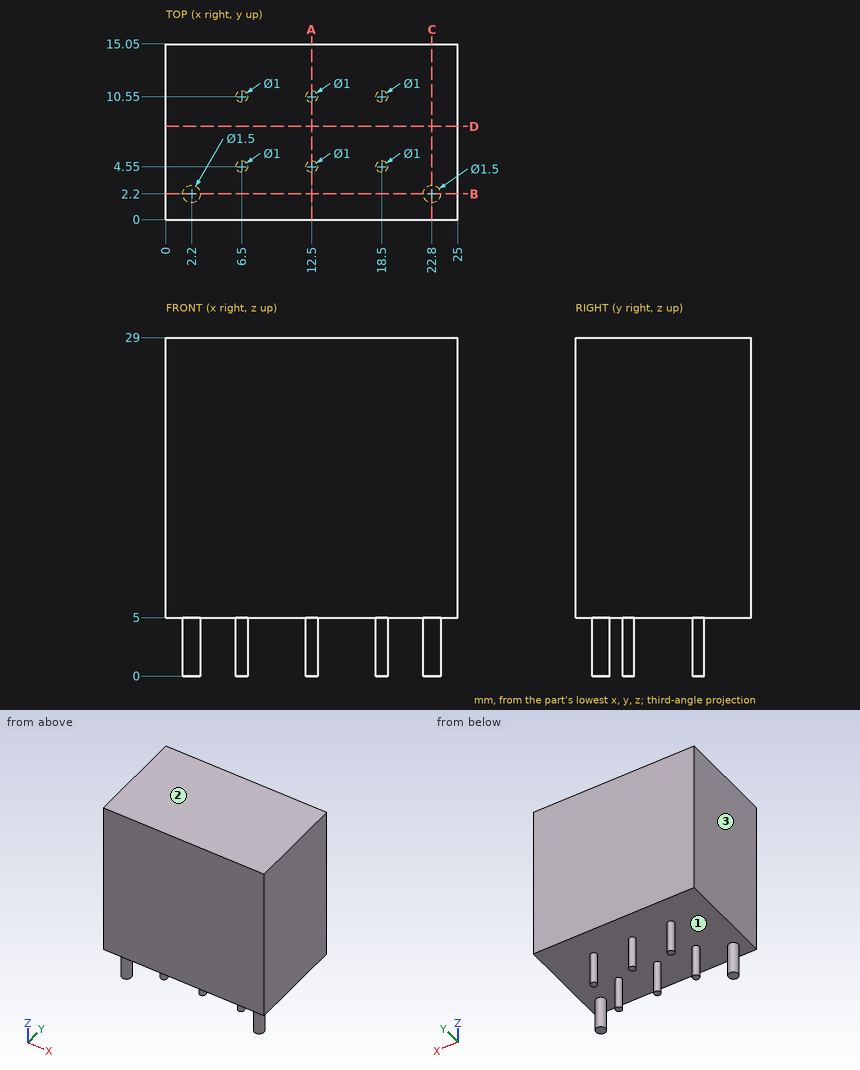
Design review of the part shown in the three views and the two pictorial views. Dimensions are in mm from the part's minimum x, y and z. Give positions to 0.01 mm unless a question says otherwise; leave off trailing zeros. Loops run counter-clockwise (first coordinate to the right, second up) from the corner with the lowest first, then second, coordinate; pieces in that order, holes last. Notation, with made-up numbers: (13, 58.25) -> (65, 58.25) arc R17 cw to (65, 76.25) -> close; hole circle Ø1 at (1, 12.5). An arc over 180 degrees is marked (long way). Answer as a JSON object with one key per item and string values. Group by question number.
Q1. Draft analysis for pull direction X (two halves, no side actions). For the marked faces 1, 2 and 3, state which applies: pulls with the +X half, pulls with the -X half, needs draft (parallel to the pull), parting line crosses it, or undercut.
Q2. Take a section at B-B (y = 2.2). Write out the cut boundary in (x, z).
Q3. Wall thickness on line 1 along Z through (x, y) = (18.75, 13): over which ranges is the line inside the solid? List them lowest first.
Q4. Take a section at C-C (x = 22.8). Write out the cut boundary in (y, z).
Q5. Take a section at A-A (x = 12.5). Write out the cut boundary in (y, z), plus the area to 3 significant figures.
Q6. Insertion check: pin 1 (6 mm diameter, centred on x = 7.5, y = 3, fed in from -Z); pin 2 (1.5 mm diameter, centred on x = 15.5, y = 2, fed in from -Z). Each pin has a flat end and moves straight along its axis. Give the tip position at first contact, or say it passes through.
Q7. Take a section at D-D (y = 8). Write out the cut boundary in (x, z), plus the area to 3 significant figures.
Answer below:
{
 "1": {"face 1": "undercut", "face 2": "needs draft", "face 3": "pulls with the -X half"},
 "2": {"outline": "(0, 5) -> (1.45, 5) -> (1.45, 0) -> (2.95, 0) -> (2.95, 5) -> (22.05, 5) -> (22.05, 0) -> (23.55, 0) -> (23.55, 5) -> (25, 5) -> (25, 29) -> (0, 29) -> close"},
 "3": {"line 1": "z = 5 to 29"},
 "4": {"outline": "(0, 5) -> (1.45, 5) -> (1.45, 0) -> (2.95, 0) -> (2.95, 5) -> (15.05, 5) -> (15.05, 29) -> (0, 29) -> close"},
 "5": {"outline": "(0, 5) -> (4.05, 5) -> (4.05, 0) -> (5.05, 0) -> (5.05, 5) -> (10.05, 5) -> (10.05, 0) -> (11.05, 0) -> (11.05, 5) -> (15.05, 5) -> (15.05, 29) -> (0, 29) -> close", "area": "371 mm2"},
 "6": {"pin 1": "stops at z = 0", "pin 2": "stops at z = 5"},
 "7": {"outline": "(0, 5) -> (25, 5) -> (25, 29) -> (0, 29) -> close", "area": "600 mm2"}
}
